Input: part model. Units: mm. Frame: model coordinates. Give positions to 0.01 mm unless a question says otherwise; leave off trailing zeros. Loops run counter-clockwise (first coordinate to the right, second up) from the corner with the lowest first, then second, coordinate; pieces in that order, holes last. Notation, with made-up numbers: (31.25, -11) -> (79.25, -11) arc R26 ccw to (79.25, 10) -> close; hole circle Ø2 at (26.5, 54). An arc over 180 degrees is marked (long way). Answer as a JSON object with one key per item and string values. Group by question number.
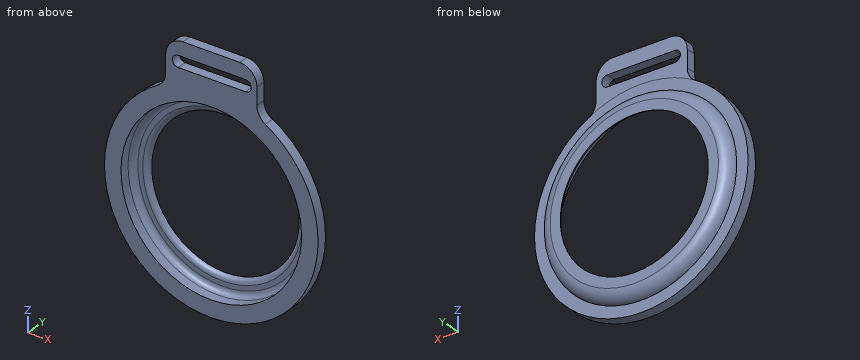
```python
from build123d import *

# Parameters (mm, degrees)
SKETCH1_R           = 18.75
BOSS_EXTRUDE1_DEPTH = 1.8
SKETCH2_R           = 16.75
BOSS_EXTRUDE2_DEPTH = 1.7
SKETCH3_R           = 13
CUT_EXTRUDE1_DEPTH  = 5.7
FILLET1_R           = 2
SKETCH4_R           = 15.85
CUT_EXTRUDE2_DEPTH  = 2.7
FILLET2_R           = 1
BOSS_EXTRUDE3_DEPTH = 1.7


with BuildPart() as part:
    # Sketch1 → Boss-Extrude1 (new body)
    with BuildSketch(Plane(origin=(0, 0, 0), x_dir=(1, 0, 0), z_dir=(0, 1, 0))):
        with Locations(Location((0, 0, 0), (0, 0, 270))):
            Circle(SKETCH1_R)
    extrude(amount=BOSS_EXTRUDE1_DEPTH)

    # Sketch2 → Boss-Extrude2 (add)
    with BuildSketch(Plane(origin=(0, 1.8, 0), x_dir=(1, 0, 0), z_dir=(0, 1, 0))):
        with Locations(Location((0, 0, 0), (0, 0, 270))):
            Circle(SKETCH2_R)
    extrude(amount=BOSS_EXTRUDE2_DEPTH)

    # Sketch3 → Cut-Extrude1 (cut)
    with BuildSketch(Plane(origin=(0, 3.5, 0), x_dir=(1, 0, 0), z_dir=(0, 1, 0))):
        with Locations(Location((0, 0, 0), (0, 0, 270))):
            Circle(SKETCH3_R)
    extrude(amount=-CUT_EXTRUDE1_DEPTH, mode=Mode.SUBTRACT)

    # Fillet1
    # the kernel refuses this fillet: 2 mm, written as the material it takes off along each edge
    with BuildSketch(Plane(origin=(0, 3.5, 0), x_dir=(0, 0, 1), z_dir=(-1, 0, 0))) as fillet1_piece_1:
        with BuildLine():
            CenterArc((14.772628007, -2), FILLET1_R, 8.626926559, 81.373073441)
            Line((14.772628007, 0), (14.772628007, 0.04))
            Line((14.772628007, 0.04), (16.75, 0.04))
            Line((16.75, 0.04), (16.79, 0))
            ThreePointArc((16.79, 0), (16.79, -0.85), (16.78954744, -1.694))
            Line((16.78954744, -1.694), (16.75, -1.7))
        make_face()
    revolve(axis=Axis((0, 3.5, 0), (0, 1, 0)), mode=Mode.SUBTRACT)

    # Sketch4 → Cut-Extrude2 (cut)
    with BuildSketch(Plane.XZ):
        with Locations(Location((0, 0, 0), (0, 0, 270))):
            Circle(SKETCH4_R)
    extrude(amount=-CUT_EXTRUDE2_DEPTH, mode=Mode.SUBTRACT)

    # Fillet2
    # the kernel refuses this fillet: 1 mm, written as the material it adds along each edge
    with BuildSketch(Plane(origin=(0, 2.7, 0), x_dir=(0, 0, -1), z_dir=(-1, 0, 0))) as fillet2_piece_1:
        with BuildLine():
            CenterArc((15.85 - FILLET2_R, FILLET2_R), FILLET2_R, 270, 90)
            Line((15.85 - FILLET2_R, 0), (15.85, 0))
            Line((15.85, 0), (15.85, FILLET2_R))
        make_face()
    revolve(axis=Axis((0, 2.7, 0), (0, -1, 0)))
    # the kernel refuses this fillet: 1 mm, written as the material it takes off along each edge
    with BuildSketch(Plane(origin=(0, 2.7, 0), x_dir=(0, 0, 1), z_dir=(-1, 0, 0))) as fillet2_2_piece_1:
        with BuildLine():
            CenterArc((13.979795897, 1), FILLET2_R, 191.536959033, 78.463040967)
            Line((13, 0.8), (13, 0))
            Line((13, 0), (13.979795897, 0))
        make_face()
    revolve(axis=Axis((0, 2.7, 0), (0, 1, 0)), mode=Mode.SUBTRACT)

    # Sketch5 → Boss-Extrude3 (add)
    with BuildSketch(Plane.XZ):
        with BuildLine():
            Line((-8, 18.763328596), (-8, 21.82057613))
            ThreePointArc((-8, 21.82057613), (-7.121320344, 23.941896474), (-5, 24.82057613))
            Line((-5, 24.82057613), (5, 24.82057613))
            ThreePointArc((5, 24.82057613), (7.121320344, 23.941896474), (8, 21.82057613))
            Line((8, 21.82057613), (8, 18.763328596))
            ThreePointArc((8, 18.763328596), (8.396951389, 17.271974201), (9.482758621, 16.175283272))
            ThreePointArc((9.482758621, 16.175283272), (0, 18.75), (-9.482758621, 16.175283272))
            ThreePointArc((-9.482758621, 16.175283272), (-8.396951389, 17.271974201), (-8, 18.763328596))
        make_face()
        with BuildLine():
            Line((-5.808489471, 22.338127717), (6.015887115, 22.338127717))
            ThreePointArc((6.015887115, 22.338127717), (7.015887115, 21.338127717), (6.015887115, 20.338127717))
            Line((6.015887115, 20.338127717), (-5.808489471, 20.338127717))
            ThreePointArc((-5.808489471, 20.338127717), (-6.808489471, 21.338127717), (-5.808489471, 22.338127717))
        make_face(mode=Mode.SUBTRACT)
    extrude(amount=-BOSS_EXTRUDE3_DEPTH)


solid = part.part
```
Q1. Section B-B on x = 0. Return the cut outline in (y, z).
Q2. Section A-A on z = 0. Return the cut outline in (x, y), then the cut area to 3 significant figures.
Q3. Ray query, probe 1 along X at (y, z) = (0.75, 0); probe 2 along Z at (x, y) = (1, 1); probe 3 along Z at (x, y) = (3, 1). Return the intervals inside material, ascending.
Q4. Pin query (flat end, axial travel): pin 1 Ø5 at (x, z) = (-9, 2.5) entering from -Y; pin 2 Ø2 at (x, y) = (8, 1) entering from -Z; pin 3 Ø0.8 at (y, z) = (1, 20) entering from -X; pin 4 Ø7 at (x, z) = (-1, 21) entering from +Y. Return the tip coordinate at first contact, or that it passes through.
Numbers:
{
 "1": {"outline": "(0, -18.75) -> (1.8, -18.75) -> (1.8, -16.75) arc R2 ccw to (3.5, -14.77) -> (3.5, -13) arc R1 ccw to (2.7, -13.98) -> (2.7, -14.85) arc R1 cw to (1.7, -15.85) -> (0, -15.85) -> close; (0, 15.85) -> (1.7, 15.85) arc R1 cw to (2.7, 14.85) -> (2.7, 13.98) arc R1 ccw to (3.5, 13) -> (3.5, 14.77) arc R2 ccw to (1.8, 16.75) -> (1.8, 18.75) -> (1.7, 18.75) -> (1.7, 20.34) -> (0, 20.34) -> close; (0, 22.34) -> (1.7, 22.34) -> (1.7, 24.82) -> (0, 24.82) -> close"},
 "2": {"outline": "(-18.75, 0) -> (-15.85, 0) -> (-15.85, 1.7) arc R1 cw to (-14.85, 2.7) -> (-13.98, 2.7) arc R1 ccw to (-13, 3.5) -> (-14.77, 3.5) arc R2 ccw to (-16.75, 1.8) -> (-18.75, 1.8) -> close; (13, 3.5) arc R1 ccw to (13.98, 2.7) -> (14.85, 2.7) arc R1 cw to (15.85, 1.7) -> (15.85, 0) -> (18.75, 0) -> (18.75, 1.8) -> (16.75, 1.8) arc R2 ccw to (14.77, 3.5) -> close", "area": "16.5 mm²"},
 "3": {"probe 1": "x = -18.75 to -15.85, 15.85 to 18.75", "probe 2": "z = -18.72 to -15.82, 15.82 to 20.34, 22.34 to 24.82", "probe 3": "z = -18.51 to -15.56, 15.56 to 20.34, 22.34 to 24.82"},
 "4": {"pin 1": "passes through", "pin 2": "stops at z = -17.39", "pin 3": "stops at x = -8", "pin 4": "stops at y = 1.8"}
}
